Can you work these out from the model? Positions are in its coordinate system, mm. Coordinates: 2 decimals unless noted, no trailing zeros. Write each loop counter-clockwise with the first axis right and the second up, starting at its lowest first coordinate (ties: lowest second). Pieces come first, ordered by that corner, then holes. Notation, with made-up numbers: (-23.75, 7) - (31.25, 7) arc R33 cw to (31.25, 45) - close; hole circle Ø9 at (-9.5, 82). An arc over 180 degrees is marked (long way). Use one line per item in the form item = value. Start each with the question number.
(1) If we section it at A-A on y = 0: Please give me the cut outline in (x, z), then the cut area to 3 significant figures.
(2) For pin 1 Ø6 at (y, z) = (-11.5, -281) entering from -X; pin 2 Ø5 at (x, z) = (1, -187.5) entering from -Y; pin 3 Ø5 at (y, z) = (-3, -294.5) entering from -X, each with a flat end and sliding along its axis, tell me the tip position at first contact or that it passes through.
(3) If we section it at C-C on z = -303.5: Please give me the cut outline in (x, y), then the cut area to 3 significant figures.
(4) If we section it at D-D on z = -443.5: Please give me the cut outline in (x, y), then the cut area to 3 significant figures.
(5) If I drill on probe 1 along Z at (x, y) = (-9.5, 17); probe 2 along Z at (x, y) = (-11, 8); probe 3 along X at (y, z) = (2, -316), over which ranges is the centre line in solid material (lowest first)? Write a range as from..to.
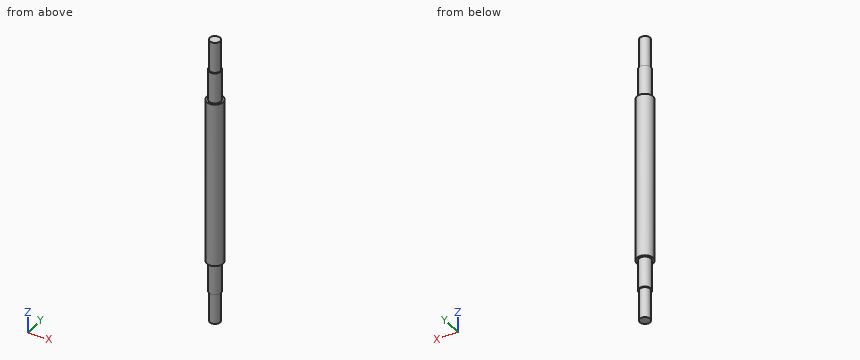
```python
from build123d import *

# Parameters (mm, degrees)
SKETCH1_R           = 20
BOSS_EXTRUDE1_DEPTH = 411.48
SKETCH2_R           = 15
BOSS_EXTRUDE2_DEPTH = 76.2
SKETCH3_R           = 15
BOSS_EXTRUDE3_DEPTH = 76.2
SKETCH4_R           = 12.7
BOSS_EXTRUDE4_DEPTH = 76.2
SKETCH5_R           = 12.7
BOSS_EXTRUDE5_DEPTH = 76.2


with BuildPart() as part:
    # Sketch1 → Boss-Extrude1 (new body)
    with BuildSketch(Plane.XY):
        Circle(SKETCH1_R)
    extrude(amount=-BOSS_EXTRUDE1_DEPTH)

    # Sketch2 → Boss-Extrude2 (add)
    with BuildSketch(Plane.XY):
        Circle(SKETCH2_R)
    extrude(amount=BOSS_EXTRUDE2_DEPTH)

    # Sketch3 → Boss-Extrude3 (add)
    with BuildSketch(Plane(origin=(0, 0, -411.48), x_dir=(-1, 0, 0), z_dir=(0, 0, -1))):
        Circle(SKETCH3_R)
    extrude(amount=BOSS_EXTRUDE3_DEPTH)

    # Sketch4 → Boss-Extrude4 (add)
    with BuildSketch(Plane.XY.offset(76.2)):
        Circle(SKETCH4_R)
    extrude(amount=BOSS_EXTRUDE4_DEPTH)

    # Sketch5 → Boss-Extrude5 (add)
    with BuildSketch(Plane(origin=(0, 0, -487.68), x_dir=(-1, 0, 0), z_dir=(0, 0, -1))):
        Circle(SKETCH5_R)
    extrude(amount=BOSS_EXTRUDE5_DEPTH)


solid = part.part
```
Reported:
q1.outline = (-20, -411.48) - (-15, -411.48) - (-15, -487.68) - (-12.7, -487.68) - (-12.7, -563.88) - (12.7, -563.88) - (12.7, -487.68) - (15, -487.68) - (15, -411.48) - (20, -411.48) - (20, 0) - (15, 0) - (15, 76.2) - (12.7, 76.2) - (12.7, 152.4) - (-12.7, 152.4) - (-12.7, 76.2) - (-15, 76.2) - (-15, 0) - (-20, 0) - close
q1.area = 24,900 mm2
q2.pin_1 = -18.1
q2.pin_2 = -20
q2.pin_3 = -19.99
q3.outline = circle Ø40 at (0, 0)
q3.area = 1,260 mm2
q4.outline = circle Ø30 at (0, 0)
q4.area = 707 mm2
q5.probe_1 = -411.48..0
q5.probe_2 = -487.68..76.2
q5.probe_3 = -19.9..19.9
